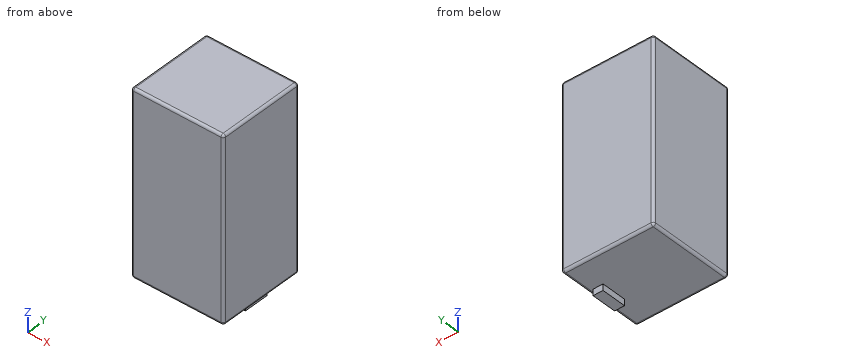
from build123d import *

# Parameters (mm, degrees)
SKETCH1_W           = 37
SKETCH1_H           = 73
BOSS_EXTRUDE1_DEPTH = 17.5
SKETCH2_W           = 4
SKETCH2_H           = 10
BOSS_EXTRUDE2_DEPTH = 2.5
FILLET1_R           = 1


with BuildPart() as part:
    # Sketch1 → Boss-Extrude1 (new body, symmetric)
    with BuildSketch(Plane(origin=(0, 0, 0), x_dir=(1, 0, 0), z_dir=(0, 1, 0))):
        Rectangle(SKETCH1_W, SKETCH1_H)
    extrude(amount=BOSS_EXTRUDE1_DEPTH, both=True)

    # Sketch2 → Boss-Extrude2 (add, symmetric)
    with BuildSketch(Plane(origin=(0, 0, -36.5), x_dir=(-1, 0, 0), z_dir=(0, 0, -1))):
        with Locations((-14.5, 0)):
            Rectangle(SKETCH2_W, SKETCH2_H)
    extrude(amount=BOSS_EXTRUDE2_DEPTH, both=True)

    # Fillet1
    fillet1_edges = [part.edges().sort_by_distance(p)[0] for p in [
        (-18.5, 17.5, 0),
        (0, 17.5, 36.5),
        (18.5, 17.5, 0),
        (0, -17.5, 36.5),
        (-18.5, -17.5, 0),
        (0, -17.5, -36.5),
        (18.5, -17.5, 0),
        (18.5, 0, 36.5),
        (-18.5, 0, 36.5),
        (-18.5, 0, -36.5),
        (18.5, 0, -36.5),
        (0, 17.5, -36.5),
    ]]
    fillet(fillet1_edges, radius=FILLET1_R)


solid = part.part
Here's how the part is built. I have some questions about the finished solid (model axes, mm). Coordinates: 2 decimals unless noted, no trailing zeros. Write each loop counter-clockwise with the first axis right and the second up, starting at its lowest first coordinate (ties: lowest second). Pieces come first, ordered by that corner, then holes.
Item 1: I want a section at A-A on y = -4. Write out the boundary of the cut face in (x, z).
Item 2: Will these pins go through, and if not, where does the flat tip stop? pin 1 (6 mm diameter, centred on x = 12.5, y = 11, fed in from -Z); pin 2 (1.2 mm diameter, centred on x = 14, z = -38.5, fed in from -Y); pin 3 (2 mm diameter, centred on x = 14, z = -37, fed in from +Y).
Item 3: I want a section at C-C on y = 13. Write out the boundary of the cut face in (x, z), and give its area (3 significant figures).
Item 4: I want a section at B-B on x = 9. Write out the boundary of the cut face in (y, z), and give its area (3 significant figures).
Item 5: If I drill on line 1 (Z direction, x = 16.5, y = 7), over which ranges is the centre line in solid material (lowest first)?
Findings below:
1. outline: (-18.5, -35.5) arc R1 ccw to (-17.5, -36.5) - (12.5, -36.5) - (12.5, -39) - (16.5, -39) - (16.5, -36.5) - (17.5, -36.5) arc R1 ccw to (18.5, -35.5) - (18.5, 35.5) arc R1 ccw to (17.5, 36.5) - (-17.5, 36.5) arc R1 ccw to (-18.5, 35.5) - close
2. pin 1: stops at z = -36.5
2. pin 2: stops at y = -5
2. pin 3: stops at y = 17.37
3. outline: (-18.5, -35.5) arc R1 ccw to (-17.5, -36.5) - (17.5, -36.5) arc R1 ccw to (18.5, -35.5) - (18.5, 35.5) arc R1 ccw to (17.5, 36.5) - (-17.5, 36.5) arc R1 ccw to (-18.5, 35.5) - close
3. area: 2,700 mm2
4. outline: (-17.5, -35.5) arc R1 ccw to (-16.5, -36.5) - (16.5, -36.5) arc R1 ccw to (17.5, -35.5) - (17.5, 35.5) arc R1 ccw to (16.5, 36.5) - (-16.5, 36.5) arc R1 ccw to (-17.5, 35.5) - close
4. area: 2,550 mm2
5. line 1: z = -36.5 to 36.5
